```python
from build123d import *

# Parameters (mm, degrees)
F0_W     = 50.8
F0_H     = 25.4
F1_DEPTH = 76.2
F2_R     = 6.35
F3_DEPTH = 6.35
F4_R     = 2.54
F5_R     = 5.08


with BuildPart() as f1:
    # F0 (on Front) → F1 (new body)
    with BuildSketch(Plane.XZ):
        with Locations((25.4, 12.7)):
            Rectangle(F0_W, F0_H)
    extrude(amount=F1_DEPTH)

    # F2 (on face) → F3 (join)
    with BuildSketch(Plane.XY.offset(25.4)):
        with Locations((25.4, -25.4)):
            Circle(F2_R)
    extrude(amount=F3_DEPTH)

    # F4
    f4_edges = [f1.edges().sort_by_distance(p)[0] for p in [
        (19.05, -25.4, 25.4),
        (19.05, -25.4, 31.75),
    ]]
    fillet(f4_edges, radius=F4_R)

    # F5
    f5_edges = [f1.edges().sort_by_distance(p)[0] for p in [
        (50.8, -76.2, 12.7),
        (50.8, 0, 12.7),
        (0, 0, 12.7),
        (0, -76.2, 12.7),
        (16.51, -25.4, 25.4),
        (50.8, -38.1, 25.4),
        (25.4, 0, 25.4),
        (25.4, -76.2, 25.4),
        (0, -38.1, 25.4),
    ]]
    fillet(f5_edges, radius=F5_R)


solid = f1.part
```
Geometry check sheet. Reference: the model listing, model coordinates, mm. A direction names the side the tool comes from. Round coordinates to 2 decimals unless told otherwise and drop trailing zeros. Order: outer loops, then holes, each group sorted by start corner. A loop starts at its lowest first (then second) coordinate and runs counter-clockwise, first axis right, second up. Notation, with made-up numbers: M 19.25,9.5 L 46.25,9.5 A30 ccw 46.25,45.5 Z; hole C 5.25,0.5 d1. An arc over 180 degrees is marked long. Write item = value, one per line.
Q1. Scan lines: line 1 (Z direction, x = 16, y = -56.5); line 2 (X direction, y = -4, z = 10.5); line 3 (X direction, y = -3.5, z = 13). Record each from-to range of solid material in increasing order.
Answer block:
line_1 = 0 to 25.4
line_2 = 0.12 to 50.68
line_3 = 0.25 to 50.55
Q2. Depth check by flat-ended pin: pin 1 Ø1.5 at (x, z) = (29, 23.5) entering from -Y; pin 2 Ø12 at (x, y) = (14.5, -43.5) entering from -Z; pin 3 Ø5 at (x, y) = (39.5, -50.5) entering from +Z. Enter the tip coordinate at first touch or a pass-through.
Answer block:
pin_1 = -75.58
pin_2 = 0
pin_3 = 25.4
Q3. Section check D-D (y = -25.4). Enter the section's corners in (x, z), plus the area to 3 significant figures.
Answer block:
outline = M 0,0 L 50.8,0 L 50.8,20.32 A5.08 ccw 45.72,25.4 L 34.29,25.4 A2.54 cw 31.75,27.94 L 31.75,29.21 A2.54 ccw 29.21,31.75 L 21.59,31.75 A2.54 ccw 19.05,29.21 L 19.05,27.94 A2.54 cw 16.51,25.4 L 5.08,25.4 A5.08 ccw 0,20.32 Z
area = 1,360 mm^2
Q4. Section check B-B (x = 44). Enter the section's corners in (y, z).
Answer block:
outline = M -76.2,0 L 0,0 L 0,20.32 A5.08 ccw -5.08,25.4 L -71.12,25.4 A5.08 ccw -76.2,20.32 Z
Q5. Section check C-C (z = 23). Enter the section's corners in (x, y), plus the area to 3 significant figures.
Answer block:
outline = M 0.76,-71.12 A4.32 ccw 5.08,-75.44 L 45.72,-75.44 A4.32 ccw 50.04,-71.12 L 50.04,-5.08 A4.32 ccw 45.72,-0.76 L 5.08,-0.76 A4.32 ccw 0.76,-5.08 Z
area = 3,660 mm^2
Q6. Section check A-A (y = -36.5). Enter the section's corners in (x, z).
Answer block:
outline = M 0,0 L 50.8,0 L 50.8,20.32 A5.08 ccw 45.72,25.4 L 5.08,25.4 A5.08 ccw 0,20.32 Z
Q7. Set-up check for faces 1 (the cylindrical face through (20.36, -29.26, 28.57)), 2 (the cylindrical face through (49, -75, 10)): record each of +Z, -Z, +X, -X, +Y, -Y from which the full face is reachable in a straight line by a thin tool's end or side.
Answer block:
face_1 = +Z
face_2 = +Z, -Z, +X, -Y
